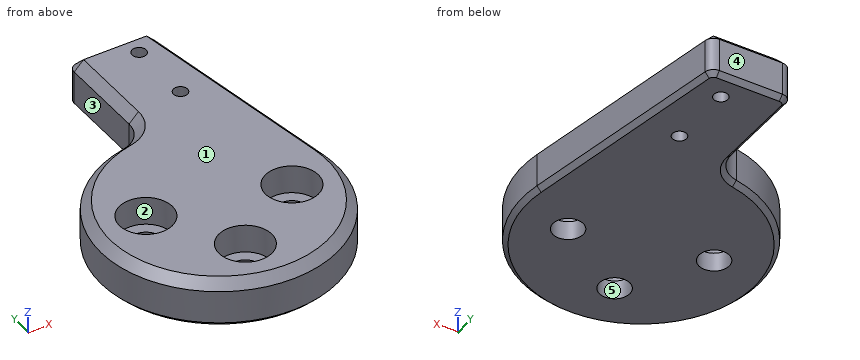
from build123d import *

# Parameters (mm, degrees)
SKETCH1_R           = 1.6
SKETCH1_R_2         = 1.6000000000000016
SKETCH1_R_3         = 0.7500000000000004
BOSS_EXTRUDE1_DEPTH = 5
CHAMFER1_SIZE       = 1
SKETCH2_R           = 2.8000000000000003
SKETCH2_R_2         = 2.8
CUT_EXTRUDE1_DEPTH  = 3
CHAMFER3_SIZE       = 0.5


with BuildPart() as part:
    # Sketch1 → Boss-Extrude1 (new body)
    with BuildSketch(Plane.XY):
        with BuildLine():
            Line((1.000000000000007, 25.491602871293395), (7.708608571885691, 25.491602871293395))
            ThreePointArc((7.708608571885691, 25.491602871293395), (8.357146361630761, 25.2527853298883), (8.695919750465407, 24.650400341838562))
            Line((8.695919750465407, 24.650400341838562), (12.341389732124407, 1.9849683817950852))
            ThreePointArc((12.341389732124407, 1.9849683817950852), (-7.1431391219536895, -10.257951232157744), (-2.41935483870505, 12.263634133540775))
            ThreePointArc((-2.41935483870505, 12.263634133540775), (-0.6824651584188808, 13.301904420618609), (-1e-17, 15.206906325619645))
            Line((-1e-17, 15.206906325619645), (-3e-17, 24.491602871293384))
            ThreePointArc((-3e-17, 24.491602871293384), (0.2928932188134522, 25.198709652479938), (1.000000000000007, 25.491602871293395))
        make_face()
        with Locations((-6.84012746585444, 1.4874999998823886)):
            Circle(SKETCH1_R, mode=Mode.SUBTRACT)
        with Locations((-1.487499999936831, -6.840127466035101)):
            Circle(SKETCH1_R, mode=Mode.SUBTRACT)
        with Locations((6.840127465980755, -1.4875000001175058)):
            Circle(SKETCH1_R_2, mode=Mode.SUBTRACT)
        with Locations((5.820860522174176, 15.749999999999972)):
            Circle(SKETCH1_R_3, mode=Mode.SUBTRACT)
        with Locations((5.820860522174148, 22.74999999999998)):
            Circle(SKETCH1_R_3, mode=Mode.SUBTRACT)
    extrude(amount=BOSS_EXTRUDE1_DEPTH)

    # Chamfer1
    chamfer1_edges = [part.edges().sort_by_distance(p)[0] for p in [
        (-0.6824651584188803, 13.301904420618609, 5),
        (-7.143139121953682, -10.25795123215775, 5),
        (10.518654741294906, 13.317684361816823, 5),
        (8.357146361630761, 25.2527853298883, 5),
        (4.354304285942849, 25.491602871293395, 5),
        (0.2928932188134533, 25.198709652479938, 5),
        (-2e-17, 19.849254598456515, 5),
    ]]
    chamfer(chamfer1_edges, length=CHAMFER1_SIZE)

    # Sketch2 → Cut-Extrude1 (cut)
    with BuildSketch(Plane.XY.offset(5)):
        with Locations((-6.84012746585444, 1.4874999998823886)):
            Circle(SKETCH2_R)
        with Locations((-1.487499999936831, -6.840127466035101)):
            Circle(SKETCH2_R_2)
        with Locations((6.840127465980755, -1.4875000001175058)):
            Circle(SKETCH2_R)
    extrude(amount=-CUT_EXTRUDE1_DEPTH, mode=Mode.SUBTRACT)

    # Chamfer3
    chamfer3_edges = [part.edges().sort_by_distance(p)[0] for p in [
        (-2e-17, 19.849254598456515, 0),
        (0.2928932188134533, 25.198709652479938, 0),
        (4.354304285942849, 25.491602871293395, 0),
        (8.357146361630761, 25.2527853298883, 0),
        (10.518654741294906, 13.317684361816823, 0),
        (-7.143139121953682, -10.25795123215775, 0),
        (-0.6824651584188803, 13.301904420618609, 0),
    ]]
    chamfer(chamfer3_edges, length=CHAMFER3_SIZE)


solid = part.part
The model under review builds one solid part; all positions refer to its coordinate system, in mm. Face numbers are marked on the shaded views. A direction names the side the tool comes from. Round coordinates to 2 decimals unless told otherwise and drop trailing zeros. Write each loop counter-clockwise with the first axis right and the second up, starting at its lowest first coordinate (ties: lowest second). Pieces come first, ordered by that corner, then holes. Notation, with made-up numbers: (2, 25.5) - (29, 25.5) arc R27 cw to (29, 48.5) - close; hole circle Ø1 at (-37.5, -38.75). An arc over 180 degrees is marked (long way). One line per item, written item: value. Start each with the question number.
1. Machinability: for the marked faces 1 and 2, which of the approach directions +Z, -Z, +X, -X, +Y, -Y give a long, thin tool a straight path to every point of the face, cutting with its end or side? Answer none if there is none.
2. To check wall thickness, follow L1, parallel to Y at x = -8.75, z = 4.55; L2, parallel to Y at x = -7.75, z = 3.25; L3, parallel to X at y = 3, z = 2.8. State the ranges of each line that lie inside material, in increasing order. Write a range as from..to.
3. Clearance check with flat-ended pins moving along their axes: P1, Ø2.5, axis at x = 5.82, y = 15.75, coming from the -Z side; P2, Ø2, axis at y = 17.5, z = 4, coming from the -X side; P3, Ø1.5, axis at x = -8, z = 2.5, coming from the -Y side; P4, Ø0.9, axis at x = 5.82, y = 22.75, coming from the +Z side. State where each tip first meets the part, or that it passes through.
4. Consider section B-B on z = 3.5. Write out the cut boundary in (x, y), and give its area (3 significant figures).
5. The part is to be moulded in two halves that separate along X. For the marked faces 3, 4 and 5, say which applies: released by +X, released by -X, zero draft, split by the parting line, or undercut.
6. Consider section C-C on y = 15.75. Write out the cut boundary in (x, z).
7. Consider section A-A on y = 22.75. Write out the cut boundary in (x, z), and give its area (3 significant figures).
Checks:
1. face 1: +Z, +X, -X, +Y, -Y
1. face 2: +Z
2. L1: y = -8.14..-0.56, 3.54..8.14
2. L2: y = -9.81..-1.16, 4.14..9.81
2. L3: x = -12.13..-9.2, -4.48..12.18
3. P1: stops at z = 0
3. P2: stops at x = 0
3. P3: stops at y = -10.18
3. P4: passes through
4. outline: (-2.42, 12.26) arc R12.5 ccw (long way) to (12.34, 1.98) - (8.7, 24.65) arc R1 ccw to (7.71, 25.49) - (1, 25.49) arc R1 ccw to (0, 24.49) - (0, 15.21) arc R3 cw to start; hole circle Ø5.6 at (-6.84, 1.49); hole circle Ø5.6 at (-1.49, -6.84); hole circle Ø5.6 at (6.84, -1.49); hole circle Ø1.5 at (5.82, 15.75); hole circle Ø1.5 at (5.82, 22.75)
4. area: 562 mm^2
5. face 3: released by -X
5. face 4: zero draft
5. face 5: undercut
6. outline: (0, 0.5) - (0.5, 0) - (5.07, 0) - (5.07, 5) - (1, 5) - (0, 4) - close; (6.57, 0) - (9.62, 0) - (10.13, 0.5) - (10.13, 4) - (9.11, 5) - (6.57, 5) - close
7. outline: (0, 0.5) - (0.5, 0) - (5.07, 0) - (5.07, 5) - (1, 5) - (0, 4) - close; (6.57, 0) - (8.5, 0) - (9, 0.5) - (9, 4) - (7.99, 5) - (6.57, 5) - close
7. area: 36.2 mm^2
